Here's how the part is built. I have some questions about the finished solid (model axes, mm). Round coordinates to 2 decimals unless told otherwise and drop trailing zeros. Write each loop counter-clockwise with the first axis right and the second up, starting at its lowest first coordinate (ties: lowest second). Pieces come first, ordered by that corner, then holes. Notation, with made-up numbers: (-7, 22) -> (-2, 22) arc R22 ccw to (-2, 35) -> close; hole circle Ø11 at (50.25, 46). An arc over 180 degrees is marked (long way). Answer in a Markdown table with one row per item. Add a question column.
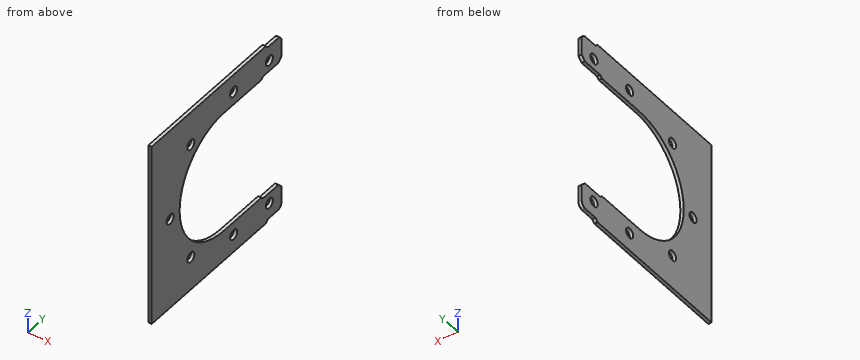
from build123d import *

# Parameters (mm, degrees)
SM_START                 = -3
SM_BASE_FLANGE_1_DEPTH   = 6
SKETCH_6_R               = 9
SKETCH_6_R_2             = 68.5
CUT_EXTRUDE_1_DEPTH      = 248.757946391
CUT_EXTRUDE_2_DEPTH      = 248.703451732
CUT_EXTRUDE_2_DEPTH_BACK = 248.703451732
FILLET_1_R               = 10
CUT_EXTRUDE_3_DEPTH      = 248.703451732
CUT_EXTRUDE_3_DEPTH_BACK = 248.703451732
SKETCH_9_W               = 4
SKETCH_9_H               = 47
CHAMFER_1_SIZE           = 8
CHAMFER_2_SIZE           = 4


# Read off the part's stored shape, not the designer's step: Базовая кромка1
with BuildPart() as part:
    # Базовая кромка1 outline → Базовая кромка1 (new body)
    with BuildSketch(Plane(origin=(0, 0, 0), x_dir=(0, 0, -1), z_dir=(1, 0, 0)).offset(SM_START)):
        with BuildLine():
            Line((-111.5, 0), (-111.5, 146))
            Line((-111.5, 146), (-168, 146))
            Line((-168, 146), (-168, -182))
            Line((-168, -182), (168, -182))
            Line((168, -182), (168, 146))
            Line((168, 146), (111.5, 146))
            Line((111.5, 146), (111.5, 0))
            ThreePointArc((111.5, 0), (0, -111.5), (-111.5, 0))
        make_face()
    extrude(amount=SM_BASE_FLANGE_1_DEPTH)

    # Эскиз6 → Вырез-Вытянуть1 (cut, through all)
    with BuildSketch(Plane(origin=(3, 0, 0), x_dir=(0, 0, -1), z_dir=(1, 0, 0))):
        with Locations((-135.25, 115)):
            Circle(SKETCH_6_R)
        with Locations((-106.578454425, -83.268214538)):
            Circle(SKETCH_6_R)
        with Locations((0, -135.25)):
            Circle(SKETCH_6_R)
        with Locations((106.578454425, -83.268214538)):
            Circle(SKETCH_6_R)
        with Locations((135.25, 115)):
            Circle(SKETCH_6_R)
        Circle(SKETCH_6_R_2)
        with Locations((-135.25, 25)):
            Circle(SKETCH_6_R)
        with Locations((135.25, 25)):
            Circle(SKETCH_6_R)
    extrude(amount=-CUT_EXTRUDE_1_DEPTH, mode=Mode.SUBTRACT)

    # Эскиз8 → Вырез-Вытянуть2 (cut, two sides: drawn at the far end of the back side and taken through both)
    with BuildSketch(Plane(origin=(0, 0, 0), x_dir=(0, 0, -1), z_dir=(1, 0, 0)).offset(-CUT_EXTRUDE_2_DEPTH_BACK)):
        Polygon((-163, 111), (-168, 106), (-168, 111), (-168, 146), (-163, 146), align=None)
        Polygon((168, 146), (163, 146), (163, 111), (168, 106), (168, 111), align=None)
    extrude(amount=CUT_EXTRUDE_2_DEPTH + CUT_EXTRUDE_2_DEPTH_BACK, mode=Mode.SUBTRACT)

    # Скругление1
    fillet_1_edges = [part.edges().sort_by_distance(p)[0] for p in [
        (0, 146, 163),
        (0, 146, -163),
    ]]
    fillet(fillet_1_edges, radius=FILLET_1_R)

    # Эскиз9 → Вырез-Вытянуть3 (cut, two sides: drawn at the far end of the back side and taken through both)
    with BuildSketch(Plane(origin=(0, 0, 0), x_dir=(0, 0, -1), z_dir=(1, 0, 0)).offset(-CUT_EXTRUDE_3_DEPTH_BACK)):
        with Locations((-113.5, 122.5)):
            Rectangle(SKETCH_9_W, SKETCH_9_H)
        with Locations((113.5, 122.5)):
            Rectangle(SKETCH_9_W, SKETCH_9_H)
    extrude(amount=CUT_EXTRUDE_3_DEPTH + CUT_EXTRUDE_3_DEPTH_BACK, mode=Mode.SUBTRACT)

    # Фаска1
    chamfer_1_edges = [part.edges().sort_by_distance(p)[0] for p in [
        (0, 146, 115.5),
        (0, 146, -115.5),
    ]]
    chamfer(chamfer_1_edges, length=CHAMFER_1_SIZE)

    # Фаска2
    chamfer_2_edges = [part.edges().sort_by_distance(p)[0] for p in [
        (0, 99, -111.5),
        (0, 99, 111.5),
    ]]
    chamfer(chamfer_2_edges, length=CHAMFER_2_SIZE - 0.0001)  # a hair under: the kernel refuses the full size


solid = part.part
Item 1: I need wall thicknesses on line 1 along Y through (x, z) = (1.45, -135.25); line 2 along Z through (x, y) = (-0.25, 114); line 3 along Z through (x, y) = (-2.25, 71.5). Which ranges of each line are inside material? Lowest first, please. Write a range as from..to.
Item 2: If we section it at A-A on y = -135.25: Please give me the cut outline in (x, z), then the cut area to 3 significant figures.
Item 3: If we section it at B-B on z = -135.25: Please give me the cut outline in (x, y), then the cut area to 3 significant figures.
Item 4: If we section it at D-D on z = 0: Please give me the cut outline in (x, y).
Item 5: For P1, Ø14.5, axis at y = 115, z = 135.25, coming from the +X side (3 decimals); P2, Ø1.8, axis at x = 0.5, y = 126.5, coming from the +Z side; P3, Ø3, axis at x = 0, y = 118.5, coming from the -Z side; P4, Ø3, axis at x = -1.5, z = 99, coming from the +Y side, each with a flat end and sliding along its axis, tell me the tip position at first contact or that it passes through.
Item 6: If we section it at C-C on y = 115: Please give me the cut outline in (x, z).
Results list:
| question | item | result |
|---|---|---|
| 1 | line 1 | -182..16, 34..106, 124..146 |
| 1 | line 2 | -163..-144.19, -126.31..-115.5, 115.5..126.31, 144.19..163 |
| 1 | line 3 | -168..-111.5, 111.5..168 |
| 2 | outline | (-3, -168) -> (3, -168) -> (3, -9) -> (-3, -9) -> close; (-3, 9) -> (3, 9) -> (3, 168) -> (-3, 168) -> close |
| 2 | area | 1,910 mm² |
| 3 | outline | (-3, -182) -> (3, -182) -> (3, 16) -> (-3, 16) -> close; (-3, 34) -> (3, 34) -> (3, 106) -> (-3, 106) -> close; (-3, 124) -> (3, 124) -> (3, 146) -> (-3, 146) -> close |
| 3 | area | 1,750 mm² |
| 4 | outline | (-3, -182) -> (3, -182) -> (3, -144.25) -> (-3, -144.25) -> close; (-3, -126.25) -> (3, -126.25) -> (3, -111.5) -> (-3, -111.5) -> close |
| 5 | P1 | through |
| 5 | P2 | z = 163 |
| 5 | P3 | z = -163 |
| 5 | P4 | y = -48.29 |
| 6 | outline | (-3, -163) -> (3, -163) -> (3, -144.25) -> (-3, -144.25) -> close; (-3, -126.25) -> (3, -126.25) -> (3, -115.5) -> (-3, -115.5) -> close; (-3, 115.5) -> (3, 115.5) -> (3, 126.25) -> (-3, 126.25) -> close; (-3, 144.25) -> (3, 144.25) -> (3, 163) -> (-3, 163) -> close |
